Check sheet for the modelled part. Datum: model origin and axes. Units: mm. A direction names the side the tool comes from. Round coordinates to 2 decimals unless told otherwise and drop trailing zeros. Write each loop counter-clockwise with the first axis right and the second up, starting at its lowest first coordinate (ties: lowest second). Pieces come first, ordered by that corner, then holes. Notation, with made-up numbers: (79.25, 54.25) -> (119.25, 54.25) arc R9 ccw to (119.25, 69.25) -> close; hole circle Ø4 at (-26.5, 76). An arc over 180 degrees is marked (long way). Use one line per item in the form item = value. Start each with the question number.
```python
from build123d import *

# Parameters (mm, degrees)
ESQUISSE1_R             = 2.5
BOSS_EXTRU_1_DEPTH      = 40
ESQUISSE2_W             = 10
ESQUISSE2_H             = 7
ENL_V_MAT_EXTRU_1_DEPTH = 44.5
ESQUISSE3_W             = 10
ESQUISSE3_H             = 8
ENL_V_MAT_EXTRU_2_DEPTH = 40
ESQUISSE4_R             = 3
ENL_V_MAT_EXTRU_3_DEPTH = 2


with BuildPart() as part:
    # Esquisse1 → Boss.-Extru.1 (new body)
    with BuildSketch(Plane(origin=(0, 0, 0), x_dir=(0, 0, -1), z_dir=(1, 0, 0))):
        with BuildLine():
            Line((-57.619622055, -2.842276543), (-20.069111797, -2.842276543))
            ThreePointArc((-20.069111797, -2.842276543), (-16.296746399, 2.898093806), (-17.619622055, -3.842276543))
            Line((-17.619622055, -3.842276543), (-57.619622055, -3.842276543))
            Line((-57.619622055, -3.842276543), (-57.619622055, -2.842276543))
        make_face()
        with Locations((-17.619622055, -0.342276543)):
            Circle(ESQUISSE1_R, mode=Mode.SUBTRACT)
    extrude(amount=BOSS_EXTRU_1_DEPTH)

    # Esquisse2 → Enlèv. mat.-Extru.1 (cut, through all)
    with BuildSketch(Plane.XY.offset(57.619622055)):
        with Locations((25, 0.657723457)):
            Rectangle(ESQUISSE2_W, ESQUISSE2_H)
        with Locations((5, 0.657723457)):
            Rectangle(ESQUISSE2_W, ESQUISSE2_H)
    extrude(amount=-ENL_V_MAT_EXTRU_1_DEPTH, mode=Mode.SUBTRACT)

    # Esquisse3 → Enlèv. mat.-Extru.2 (cut)
    with BuildSketch(Plane(origin=(0, -2.842276543, 0), x_dir=(1, 0, 0), z_dir=(0, 1, 0))):
        with Locations((5, -18.119622055)):
            Rectangle(ESQUISSE3_W, ESQUISSE3_H)
        with Locations((25, -18.119622055)):
            Rectangle(ESQUISSE3_W, ESQUISSE3_H)
    extrude(amount=-ENL_V_MAT_EXTRU_2_DEPTH, mode=Mode.SUBTRACT)

    # Esquisse4 → Enlèv. mat.-Extru.3 (cut, through all)
    with BuildSketch(Plane(origin=(0, -2.842276543, 0), x_dir=(1, 0, 0), z_dir=(0, 1, 0))):
        with Locations(Location((10, -37.619622055, 0), (0, 0, 270))):  # turned: the seam where the file's is
            Circle(ESQUISSE4_R)
        with Locations(Location((20, -37.619622055, 0), (0, 0, 270))):  # turned: the seam where the file's is
            Circle(ESQUISSE4_R)
        with Locations(Location((30, -37.619622055, 0), (0, 0, 270))):  # turned: the seam where the file's is
            Circle(ESQUISSE4_R)
        with BuildLine():
            Line((10, -47.619622055), (30, -47.619622055))
            ThreePointArc((30, -47.619622055), (37.071067812, -44.690689866), (40, -37.619622055))
            Line((40, -37.619622055), (40, -57.619622055))
            Line((40, -57.619622055), (0, -57.619622055))
            Line((0, -57.619622055), (0, -37.619622055))
            ThreePointArc((0, -37.619622055), (2.928932188, -44.690689866), (10, -47.619622055))
        make_face()
    extrude(amount=-ENL_V_MAT_EXTRU_3_DEPTH, mode=Mode.SUBTRACT)


solid = part.part
```
1. Tool access check on faces 4 (the face through (30, -3, 19)), 5 (the face through (5, -3, 22.12)), 6 (the face through (40, -3, 23)). Record the directions out of +Z, -Z, +X, -X, +Y, -Y that give a thin tool (end or side, any length) a straight path to the whole face; none if there is none.
2. Sectioned sample at C-C (z = 38.5). Enter the section's corners in (x, y), and give its area (3 significant figures).
3. Sectioned sample at D-D (x = 15). Enter the section's corners in (y, z), and give its area (3 significant figures).
4. Depth check by flat-ended pin: pin 1 (4 mm diameter, centred on y = -0.34, z = 17.62, fed in from +X); pin 2 (8 mm diameter, centred on x = 20, z = 37.62, fed in from +Y); pin 3 (1 mm diameter, centred on x = 15.5, z = 21, fed in from +Y); pin 4 (1 mm diameter, centred on x = 31, y = -2, fed in from -Z). Enter the tip coordinate at first touch or a pass-through.
5. Scan lines: probe 1 along X at (y, z) = (-3.5, 21); probe 2 along Y at (x, z) = (35, 44.5); probe 3 along Z at (x, y) = (15.5, 0). Record each from-to range of solid material in increasing order.
6. Mould release check, pull along Y, two halves, no side actions. Record for faces 1 (the face through (34.93, 0.409, 15.235)), 2 (the face through (20, -3.842, 32)), 3 (the face through (25, -3, 22.12)): +Y half, -Y half, draft (parallel to the pull), parting line (faces both ways), or undercut.
7. Sectioned sample at A-A (y = -1.75). Enter the section's corners in (x, z), and give its area (3 significant figures).
8. Sectioned sample at B-B (x = 29). Enter the section's corners in (y, z), and give its area (3 significant figures).
Returned:
q1.face_4 = -Z, +Y, -Y
q1.face_5 = -Z, -X, +Y, -Y
q1.face_6 = +Z, -Z, +X, +Y, -Y
q2.outline = (0.04, -3.84) -> (7.13, -3.84) -> (7.13, -2.84) -> (0.04, -2.84) -> close; (12.87, -3.84) -> (17.13, -3.84) -> (17.13, -2.84) -> (12.87, -2.84) -> close; (22.87, -3.84) -> (27.13, -3.84) -> (27.13, -2.84) -> (22.87, -2.84) -> close; (32.87, -3.84) -> (39.96, -3.84) -> (39.96, -2.84) -> (32.87, -2.84) -> close
q2.area = 22.7 mm^2
q3.outline = (-3.84, 17.62) arc R3.5 ccw (long way) to (-2.84, 20.07) -> (-2.84, 47.62) -> (-3.84, 47.62) -> close; hole circle Ø5 at (-0.34, 17.62)
q3.area = 47.2 mm^2
q4.pin_1 = through
q4.pin_2 = -2.84
q4.pin_3 = 1.65
q4.pin_4 = 14.32
q5.probe_1 = 10 to 20, 30 to 40
q5.probe_2 = -3.84 to -2.84
q5.probe_3 = 14.14 to 15.14, 20.1 to 21.1
q6.face_1 = undercut
q6.face_2 = -Y half
q6.face_3 = draft
q7.outline = (10, 14.42) -> (20, 14.42) -> (20, 15.55) -> (10, 15.55) -> close; (10, 19.69) -> (20, 19.69) -> (20, 20.82) -> (10, 20.82) -> close; (30, 14.42) -> (40, 14.42) -> (40, 15.55) -> (30, 15.55) -> close; (30, 19.69) -> (40, 19.69) -> (40, 20.82) -> (30, 20.82) -> close
q7.area = 45.5 mm^2
q8.outline = (-3.84, 22.12) -> (-2.84, 22.12) -> (-2.84, 34.79) -> (-3.84, 34.79) -> close; (-3.84, 40.45) -> (-2.84, 40.45) -> (-2.84, 47.62) -> (-3.84, 47.62) -> close
q8.area = 19.8 mm^2
